Model file for the job. Use its own axes, mm. A direction names the side the tool comes from. Round coordinates to 2 decimals unless told otherwise and drop trailing zeros. Loops run counter-clockwise (first coordinate to the right, second up) from the corner with the lowest first, then second, coordinate; pieces in that order, holes last. Notation, with made-up numbers: (32.5, 26.5) -> (42.5, 26.5) arc R30 ccw to (42.5, 56.5) -> close; hole circle Ø2 at (83.25, 73.25). An arc over 180 degrees is marked (long way). Use a Markdown table: item, result.
from build123d import *

# Parameters (mm, degrees)
SKETCH1_R           = 50
BOSS_EXTRUDE1_DEPTH = 25
SKETCH2_R           = 32.625
CUT_EXTRUDE1_DEPTH  = 6.75
SKETCH3_W           = 23.5
SKETCH3_H           = 23.5
CUT_EXTRUDE2_DEPTH  = 4.3
CUT_EXTRUDE3_DEPTH  = 13.95
SKETCH24_W          = 23.5
SKETCH24_H          = 23.5
CUT_EXTRUDE4_DEPTH  = 11
SKETCH25_R          = 50
CUT_EXTRUDE5_DEPTH  = 7
SKETCH26_R          = 1.2
CUT_EXTRUDE6_DEPTH  = 72.568865437
BOSS_EXTRUDE2_START = 7.5
BOSS_EXTRUDE2_DEPTH = 7.5


with BuildPart() as part:
    # Sketch1 → Boss-Extrude1 (new body)
    with BuildSketch(Plane(origin=(0, 0, 0), x_dir=(1, 0, 0), z_dir=(0, 1, 0))):
        with Locations(Location((0, 0, 0), (0, 0, 270))):
            Circle(SKETCH1_R)
    extrude(amount=BOSS_EXTRUDE1_DEPTH)

    # Sketch2 → Cut-Extrude1 (cut)
    with BuildSketch(Plane(origin=(0, 25, 0), x_dir=(1, 0, 0), z_dir=(0, 1, 0))):
        with Locations(Location((0, 0, 0), (0, 0, 270))):
            Circle(SKETCH2_R)
    extrude(amount=-CUT_EXTRUDE1_DEPTH, mode=Mode.SUBTRACT)

    # Sketch3 → Cut-Extrude2 (cut)
    with BuildSketch(Plane(origin=(0, 18.25, 0), x_dir=(1, 0, 0), z_dir=(0, 1, 0))):
        Rectangle(SKETCH3_W, SKETCH3_H)
    extrude(amount=-CUT_EXTRUDE2_DEPTH, mode=Mode.SUBTRACT)

    # Sketch4 → Cut-Extrude3 (cut)
    with BuildSketch(Plane(origin=(0, 13.95, 0), x_dir=(1, 0, 0), z_dir=(0, 1, 0))):
        with BuildLine():
            Line((-11.75, 4.95), (-7.1, 4.95))
            ThreePointArc((-7.1, 4.95), (-5.525793851, 5.571198073), (-4.8, 7.1))
            Line((-4.8, 7.1), (-4.8, 11.75))
            Line((-4.8, 11.75), (11.75, 11.75))
            Line((11.75, 11.75), (11.75, -4.8))
            Line((11.75, -4.8), (7.1, -4.8))
            ThreePointArc((7.1, -4.8), (5.571198073, -5.525793851), (4.95, -7.1))
            Line((4.95, -7.1), (4.95, -11.75))
            Line((4.95, -11.75), (-11.75, -11.75))
            Line((-11.75, -11.75), (-11.75, 4.95))
        make_face()
    extrude(amount=-CUT_EXTRUDE3_DEPTH, mode=Mode.SUBTRACT)

    # Sketch24 → Cut-Extrude4 (cut)
    with BuildSketch(Plane.XZ):
        Rectangle(SKETCH24_W, SKETCH24_H)
    extrude(amount=-CUT_EXTRUDE4_DEPTH, mode=Mode.SUBTRACT)

    # Sketch25 → Cut-Extrude5 (cut)
    with BuildSketch(Plane.XZ):
        with Locations(Location((0, 0, 0), (0, 0, 270))):
            Circle(SKETCH25_R)
    extrude(amount=-CUT_EXTRUDE5_DEPTH, mode=Mode.SUBTRACT)

    # Sketch26 → Cut-Extrude6 (cut, through all)
    with BuildSketch(Plane(origin=(0, 13.95, 0), x_dir=(1, 0, 0), z_dir=(0, 1, 0))):
        with Locations(Location((-7.638603897, 7.713603897, 0), (0, 0, 270))):
            Circle(SKETCH26_R)
        with Locations(Location((7.713603897, -7.638603897, 0), (0, 0, 270))):
            Circle(SKETCH26_R)
    extrude(amount=-CUT_EXTRUDE6_DEPTH, mode=Mode.SUBTRACT)

    # Sketch27 → Boss-Extrude2 (add)
    with BuildSketch(Plane.XZ.offset(-7).offset(BOSS_EXTRUDE2_START)):
        with BuildLine():
            Line((-50, 0), (-40, 0))
            ThreePointArc((-40, 0), (-28.284271247, 28.284271247), (0, 40))
            Line((0, 40), (0, 50))
            ThreePointArc((0, 50), (-35.355339059, 35.355339059), (-50, 0))
        make_face()
        with BuildLine():
            Line((40, 0), (50, 0))
            ThreePointArc((50, 0), (35.355339059, -35.355339059), (0, -50))
            Line((0, -50), (0, -40))
            ThreePointArc((0, -40), (28.284271247, -28.284271247), (40, 0))
        make_face()
    extrude(amount=-BOSS_EXTRUDE2_DEPTH)


solid = part.part
Q1. Band-saw the part on B-B, the plane x = -2. Give the cut face in (y, z).
Results list:
| item | result |
|---|---|
| outline | (-0.5, 39.95) -> (7, 39.95) -> (7, 11.75) -> (18.25, 11.75) -> (18.25, 32.56) -> (25, 32.56) -> (25, 49.96) -> (-0.5, 49.96) -> close; (7, -49.96) -> (25, -49.96) -> (25, -32.56) -> (18.25, -32.56) -> (18.25, -11.75) -> (7, -11.75) -> close |
Q2. Band-saw the part on C-C, the plane y = 16.5. Give the cut face in (x, z), plus the area to 3 significant figures.
Results list:
| item | result |
|---|---|
| outline | circle Ø100 at (0, 0); hole (-11.75, -11.75) -> (11.75, -11.75) -> (11.75, 11.75) -> (-11.75, 11.75) -> close |
| area | 7,300 mm² |
Q3. Flat gauge pins, fed straight in: pin 1 (10 mm diameter, centred on y = 21, z = -0.5, fed in from +X); pin 2 (8 mm diameter, centred on x = 44, y = 2.5, fed in from +Z); pin 3 (19.5 mm diameter, centred on x = -2, z = 11, fed in from +Y); pin 4 (1.4 mm diameter, centred on x = -7.64, z = -7.71, fed in from +Y). Where does each tip first touch, or does it go through?
Results list:
| item | result |
|---|---|
| pin 1 | stops at x = 50 |
| pin 2 | stops at z = 0 |
| pin 3 | stops at y = 18.25 |
| pin 4 | passes through |
Q4. Band-saw the part on D-D, the plane z = 29.5. Give the cut face in (x, y).
Results list:
| item | result |
|---|---|
| outline | (-40.37, -0.5) -> (-27.01, -0.5) -> (-27.01, 7) -> (40.37, 7) -> (40.37, 25) -> (13.93, 25) -> (13.93, 18.25) -> (-13.93, 18.25) -> (-13.93, 25) -> (-40.37, 25) -> close |
Q5. Band-saw the part on A-A, the plane y = 5. Give the cut face in (x, z).
Results list:
| item | result |
|---|---|
| outline | (-50, 0) -> (-40, 0) arc R40 cw to (0, 40) -> (0, 50) arc R50 ccw to start; (0, -50) arc R50 ccw to (50, 0) -> (40, 0) arc R40 cw to (0, -40) -> close |
Q6. Tool access for faces 5 (the face through (-8.3, 11, -9.1)), 6 (the face through (0, 18.25, 14)), 7 (the face through (9, 12, 4.8)), 8 (the face through (45, 3, 0)), 9 (the face through (11.75, 13, 0)): list every direction of +Z, -Z, +X, -X, +Y, -Y with a clear straight run to the whole face (end or side of a thin tool).
Results list:
| item | result |
|---|---|
| face 5 | -Y |
| face 6 | +Y |
| face 7 | +Y, -Y |
| face 8 | +Z, +X, -Y |
| face 9 | none |
Q7. Drill centre lines: L1, parallel to X at y = 23.25, z = 0 (3 decimals); L2, parallel to Y at x = -21.5, z = -36.5; L3, parallel to X at y = 20.25, z = -25. Where is each one in solid material? Low to high. Write a range as from..to.
Results list:
| item | result |
|---|---|
| L1 | x = -50..-32.625, 32.625..50 |
| L2 | y = 7..25 |
| L3 | x = -43.3..-20.96, 20.96..43.3 |
Q8. Pull direction X, two halves, no side cores. Call faces 1 (the face through (-28.594, 3.198, 27.972)), 2 (the face through (1, 25, 33)), 3 (the face through (0, 3, -45)), 4 (the face through (0, 13, 11.75)): released by +X, released by -X, zero draft, split by the parting line, or undercut.
Results list:
| item | result |
|---|---|
| face 1 | released by +X |
| face 2 | zero draft |
| face 3 | released by -X |
| face 4 | undercut |
